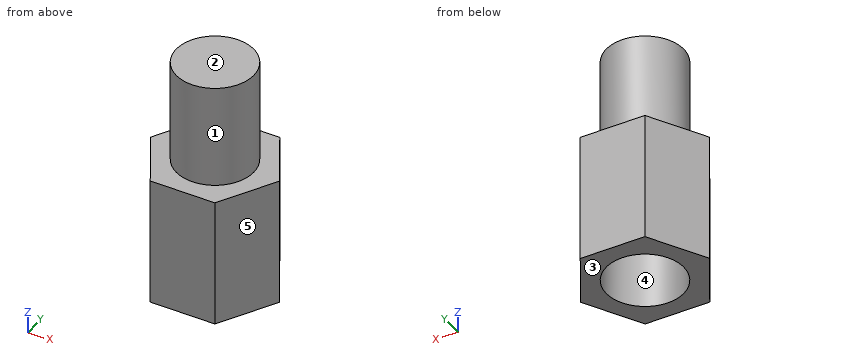
```python
from build123d import *

# Parameters (mm, degrees)
F1_DEPTH = 5
F2_R     = 1.5
F3_DEPTH = 4
F4_R     = 1.5
F5_DEPTH = 4


with BuildPart() as f1:
    # F0 (on Top) → F1 (new body)
    with BuildSketch(Plane.XY):
        Polygon((1.25, -2.165064), (2.5, 0), (1.25, 2.165064), (-1.25, 2.165064), (-2.5, 0), (-1.25, -2.165064), align=None)
    extrude(amount=F1_DEPTH)

    # F2 (on face) → F3 (join)
    with BuildSketch(Plane.XY.offset(5)):
        Circle(F2_R)
    extrude(amount=F3_DEPTH)

    # F4 (on face) → F5 (cut)
    with BuildSketch(Plane.XY):
        Circle(F4_R)
    extrude(amount=F5_DEPTH, mode=Mode.SUBTRACT)


solid = f1.part
```
Could you check a few things on this model? Use its own coordinates, in mm. Face numbers are marked on the shaded views. A direction names the side the tool comes from. Round coordinates to 2 decimals unless told otherwise and drop trailing zeros. Loops run counter-clockwise (first coordinate to the right, second up) from the corner with the lowest first, then second, coordinate; pieces in that order, holes last.
Q1. Thinking about a two-plate mould opening in X: for the marked faces 3, 4 and 5, which applies, pulls with the +X half, pulls with the -X half, needs draft (parallel to the pull), parting line crosses it, or undercut?
Q2. I want a section at D-D (y = -0.5). Write out the boundary of the cut face in (x, z), and give its area (3 significant figures).
Q3. I want a section at C-C (z = 4.75). Write out the boundary of the cut face in (x, y).
Q4. I want a section at B-B (x = 0). Write out the boundary of the cut face in (y, z).
Q5. I want a section at A-A (z = 1.25). Write out the boundary of the cut face in (x, y).
Q6. Please list where these lines run through material, in increasing order: L1, parallel to Y at x = 0, z = 2.3; L2, parallel to Z at x = 0.5, y = -0.7; L3, parallel to Z at x = -1.35, y = 1.2.
Q7. For P1, Ø1, axis at x = 2, y = -0.5, coming from the +Z side; P2, Ø1, axis at y = -1, z = 1, coming from the +X side; P3, Ø2, axis at y = -1.5, z = 7.5, coming from the +X side, each with a flat end and sliding along its axis, tell me the tip position at first contact or that it passes through.
Q8. On a 3-axis mill with a long thin cutter (end or side, diameter ignored), from which of +Z, -Z, +X, -X, +Y, -Y can I reach the whole of each face in a straight line? I mean the marked faces 1 and 2. Say none if no direction works.
Answer below:
1. face 3: needs draft
1. face 4: undercut
1. face 5: pulls with the +X half
2. outline: (-2.21, 0) - (-1.41, 0) - (-1.41, 4) - (1.41, 4) - (1.41, 0) - (2.21, 0) - (2.21, 5) - (1.41, 5) - (1.41, 9) - (-1.41, 9) - (-1.41, 5) - (-2.21, 5) - close
2. area: 22.1 mm2
3. outline: (-2.5, 0) - (-1.25, -2.17) - (1.25, -2.17) - (2.5, 0) - (1.25, 2.17) - (-1.25, 2.17) - close
4. outline: (-2.17, 0) - (-1.5, 0) - (-1.5, 4) - (1.5, 4) - (1.5, 0) - (2.17, 0) - (2.17, 5) - (1.5, 5) - (1.5, 9) - (-1.5, 9) - (-1.5, 5) - (-2.17, 5) - close
5. outline: (-2.5, 0) - (-1.25, -2.17) - (1.25, -2.17) - (2.5, 0) - (1.25, 2.17) - (-1.25, 2.17) - close; hole circle Ø3 at (0, 0)
6. L1: y = -2.17 to -1.5, 1.5 to 2.17
6. L2: z = 4 to 9
6. L3: z = 0 to 5
7. P1: stops at z = 5
7. P2: stops at x = 2.21
7. P3: stops at x = 1.41
8. face 1: +Z
8. face 2: +Z, +X, -X, +Y, -Y
